from build123d import *

# Parameters (mm, degrees)
BOSS_EXTRUDE1_DEPTH = 280
SKETCH5_W           = 95
SKETCH5_H           = 160
SKETCH5_W_2         = 95.780958046
CUT_EXTRUDE9_DEPTH  = 280
FILLET1_RADIUS      = 30
FILLET1_LENGTH      = 15
FILLET2_RADIUS      = 30
FILLET2_LENGTH      = 15
FILLET3_RADIUS      = 30
FILLET3_LENGTH      = 15
FILLET4_RADIUS      = 30
FILLET4_LENGTH      = 15
SKETCH7_R           = 15
CUT_EXTRUDE10_DEPTH = 280
SKETCH8_W           = 140
SKETCH8_H           = 61.010205144
CUT_EXTRUDE11_DEPTH = 280
FILLET5_RADIUS      = 35
FILLET5_LENGTH      = 15
FILLET6_RADIUS      = 35
FILLET6_LENGTH      = 15
FILLET7_RADIUS      = 35
FILLET7_LENGTH      = 15
FILLET8_RADIUS      = 35
FILLET8_LENGTH      = 15
SKETCH9_R           = 15
CUT_EXTRUDE12_DEPTH = 280


with BuildPart() as part:
    # Sketch1 → Boss-Extrude1 (new body)
    with BuildSketch(Plane.XY):
        with BuildLine():
            Line((-120, -40), (-37.749172176, -40))
            ThreePointArc((-37.749172176, -40), (-54.444104817, 7.799964787), (-25, 48.989794856))
            Line((-25, 48.989794856), (-25, 110))
            Line((-25, 110), (-10, 110))
            Line((-10, 110), (-10, 38.729833462))
            ThreePointArc((-10, 38.729833462), (0, -40), (10, 38.729833462))
            Line((10, 38.729833462), (10, 110))
            Line((10, 110), (25, 110))
            Line((25, 110), (25, 48.989794856))
            ThreePointArc((25, 48.989794856), (54.444104817, 7.799964787), (37.749172176, -40))
            Line((37.749172176, -40), (120, -40))
            Line((120, -40), (120, -55))
            Line((120, -55), (-120, -55))
            Line((-120, -55), (-120, -40))
        make_face()
    extrude(amount=-BOSS_EXTRUDE1_DEPTH)

    # Sketch5 → Cut-Extrude9 (cut)
    with BuildSketch(Plane(origin=(0, -40, 0), x_dir=(1, 0, 0), z_dir=(0, 1, 0))):
        with Locations((72.5, 140)):
            Rectangle(SKETCH5_W, SKETCH5_H)
        with Locations((-72.109520977, 140)):
            Rectangle(SKETCH5_W_2, SKETCH5_H)
    extrude(amount=-CUT_EXTRUDE9_DEPTH, mode=Mode.SUBTRACT)

    # Fillet1: full round fillet: the end face becomes a half cylinder, R = half its width
    fillet1_face = Plane((-120, -47.5, -250), x_dir=(0, -1, 0), z_dir=(-1, 0, 0))  # on the end face: x along it, z out of the body
    fillet1_slab = fillet1_face.offset(-FILLET1_RADIUS / 2) * Box(FILLET1_LENGTH, 2 * FILLET1_RADIUS, FILLET1_RADIUS, mode=Mode.PRIVATE)  # the body's end, R deep
    fillet1_round = Plane((-90, -47.5, -250), x_dir=(-1, 0, 0), z_dir=(0, -1, 0)) * Cylinder(FILLET1_RADIUS, FILLET1_LENGTH, mode=Mode.PRIVATE)  # its axis R under the face
    add(fillet1_slab - fillet1_round, mode=Mode.SUBTRACT)

    # Fillet2: full round fillet: the end face becomes a half cylinder, R = half its width
    fillet2_face = Plane((-120, -47.5, -30), x_dir=(0, 1, 0), z_dir=(-1, 0, 0))  # on the end face: x along it, z out of the body
    fillet2_slab = fillet2_face.offset(-FILLET2_RADIUS / 2) * Box(FILLET2_LENGTH, 2 * FILLET2_RADIUS, FILLET2_RADIUS, mode=Mode.PRIVATE)  # the body's end, R deep
    fillet2_round = Plane((-90, -47.5, -30), x_dir=(-1, 0, 0), z_dir=(0, 1, 0)) * Cylinder(FILLET2_RADIUS, FILLET2_LENGTH, mode=Mode.PRIVATE)  # its axis R under the face
    add(fillet2_slab - fillet2_round, mode=Mode.SUBTRACT)

    # Fillet3: full round fillet: the end face becomes a half cylinder, R = half its width
    fillet3_face = Plane((120, -47.5, -250), x_dir=(0, 1, 0), z_dir=(1, 0, 0))  # on the end face: x along it, z out of the body
    fillet3_slab = fillet3_face.offset(-FILLET3_RADIUS / 2) * Box(FILLET3_LENGTH, 2 * FILLET3_RADIUS, FILLET3_RADIUS, mode=Mode.PRIVATE)  # the body's end, R deep
    fillet3_round = Plane((90, -47.5, -250), x_dir=(1, 0, 0), z_dir=(0, 1, 0)) * Cylinder(FILLET3_RADIUS, FILLET3_LENGTH, mode=Mode.PRIVATE)  # its axis R under the face
    add(fillet3_slab - fillet3_round, mode=Mode.SUBTRACT)

    # Fillet4: full round fillet: the end face becomes a half cylinder, R = half its width
    fillet4_face = Plane((120, -47.5, -30), x_dir=(0, -1, 0), z_dir=(1, 0, 0))  # on the end face: x along it, z out of the body
    fillet4_slab = fillet4_face.offset(-FILLET4_RADIUS / 2) * Box(FILLET4_LENGTH, 2 * FILLET4_RADIUS, FILLET4_RADIUS, mode=Mode.PRIVATE)  # the body's end, R deep
    fillet4_round = Plane((90, -47.5, -30), x_dir=(1, 0, 0), z_dir=(0, -1, 0)) * Cylinder(FILLET4_RADIUS, FILLET4_LENGTH, mode=Mode.PRIVATE)  # its axis R under the face
    add(fillet4_slab - fillet4_round, mode=Mode.SUBTRACT)

    # Sketch7 → Cut-Extrude10 (cut)
    with BuildSketch(Plane(origin=(0, -40, 0), x_dir=(1, 0, 0), z_dir=(0, 1, 0))):
        with Locations(Location((-90, 250, 0), (0, 0, 180))):
            Circle(SKETCH7_R)
        with Locations(Location((90, 250, 0), (0, 0, 180))):
            Circle(SKETCH7_R)
        with Locations(Location((90, 30, 0), (0, 0, 180))):
            Circle(SKETCH7_R)
        with Locations(Location((-90, 30, 0), (0, 0, 180))):
            Circle(SKETCH7_R)
    extrude(amount=-CUT_EXTRUDE10_DEPTH, mode=Mode.SUBTRACT)

    # Sketch8 → Cut-Extrude11 (cut)
    with BuildSketch(Plane(origin=(25, 0, 0), x_dir=(0, 0, -1), z_dir=(1, 0, 0))):
        with Locations((140, 79.494897428)):
            Rectangle(SKETCH8_W, SKETCH8_H)
    extrude(amount=-CUT_EXTRUDE11_DEPTH, mode=Mode.SUBTRACT)

    # Fillet5: full round fillet: the end face becomes a half cylinder, R = half its width
    fillet5_face = Plane((17.5, 110, -35), x_dir=(1, 0, 0), z_dir=(0, 1, 0))  # on the end face: x along it, z out of the body
    fillet5_slab = fillet5_face.offset(-FILLET5_RADIUS / 2) * Box(FILLET5_LENGTH, 2 * FILLET5_RADIUS, FILLET5_RADIUS, mode=Mode.PRIVATE)  # the body's end, R deep
    fillet5_round = Plane((17.5, 75, -35), x_dir=(0, 1, 0), z_dir=(1, 0, 0)) * Cylinder(FILLET5_RADIUS, FILLET5_LENGTH, mode=Mode.PRIVATE)  # its axis R under the face
    add(fillet5_slab - fillet5_round, mode=Mode.SUBTRACT)

    # Fillet6: full round fillet: the end face becomes a half cylinder, R = half its width
    fillet6_face = Plane((-17.5, 110, -35), x_dir=(1, 0, 0), z_dir=(0, 1, 0))  # on the end face: x along it, z out of the body
    fillet6_slab = fillet6_face.offset(-FILLET6_RADIUS / 2) * Box(FILLET6_LENGTH, 2 * FILLET6_RADIUS, FILLET6_RADIUS, mode=Mode.PRIVATE)  # the body's end, R deep
    fillet6_round = Plane((-17.5, 75, -35), x_dir=(0, 1, 0), z_dir=(1, 0, 0)) * Cylinder(FILLET6_RADIUS, FILLET6_LENGTH, mode=Mode.PRIVATE)  # its axis R under the face
    add(fillet6_slab - fillet6_round, mode=Mode.SUBTRACT)

    # Fillet7: full round fillet: the end face becomes a half cylinder, R = half its width
    fillet7_face = Plane((-17.5, 110, -245), x_dir=(1, 0, 0), z_dir=(0, 1, 0))  # on the end face: x along it, z out of the body
    fillet7_slab = fillet7_face.offset(-FILLET7_RADIUS / 2) * Box(FILLET7_LENGTH, 2 * FILLET7_RADIUS, FILLET7_RADIUS, mode=Mode.PRIVATE)  # the body's end, R deep
    fillet7_round = Plane((-17.5, 75, -245), x_dir=(0, 1, 0), z_dir=(1, 0, 0)) * Cylinder(FILLET7_RADIUS, FILLET7_LENGTH, mode=Mode.PRIVATE)  # its axis R under the face
    add(fillet7_slab - fillet7_round, mode=Mode.SUBTRACT)

    # Fillet8: full round fillet: the end face becomes a half cylinder, R = half its width
    fillet8_face = Plane((17.5, 110, -245), x_dir=(1, 0, 0), z_dir=(0, 1, 0))  # on the end face: x along it, z out of the body
    fillet8_slab = fillet8_face.offset(-FILLET8_RADIUS / 2) * Box(FILLET8_LENGTH, 2 * FILLET8_RADIUS, FILLET8_RADIUS, mode=Mode.PRIVATE)  # the body's end, R deep
    fillet8_round = Plane((17.5, 75, -245), x_dir=(0, 1, 0), z_dir=(1, 0, 0)) * Cylinder(FILLET8_RADIUS, FILLET8_LENGTH, mode=Mode.PRIVATE)  # its axis R under the face
    add(fillet8_slab - fillet8_round, mode=Mode.SUBTRACT)

    # Sketch9 → Cut-Extrude12 (cut)
    with BuildSketch(Plane(origin=(25, 0, 0), x_dir=(0, 0, -1), z_dir=(1, 0, 0))):
        with Locations((35, 75)):
            Circle(SKETCH9_R)
        with Locations((245, 75)):
            Circle(SKETCH9_R)
    extrude(amount=-CUT_EXTRUDE12_DEPTH, mode=Mode.SUBTRACT)


solid = part.part
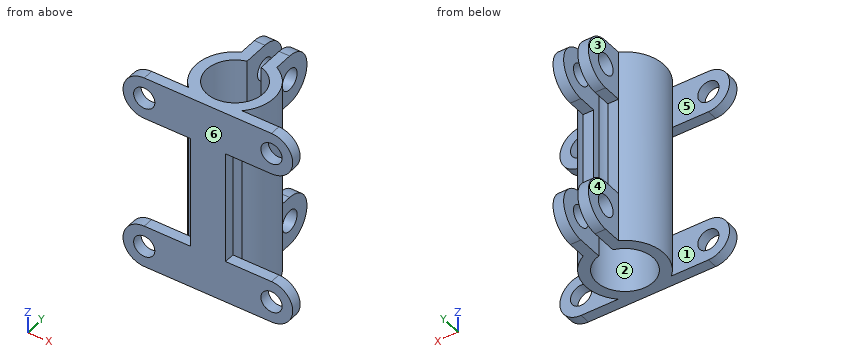
Source: CAD feature listing. Evaluate the final solid. Frame: model axes, mm. Face numbers are marked on the shaded views. A direction names the side the tool comes from. Give positions to 0.01 mm unless a question says otherwise; leave off trailing zeros. Order: outer loops, then holes, each group sorted by start corner. A loop starts at its lowest first (then second) coordinate and runs counter-clockwise, first axis right, second up. Notation, with made-up numbers: (16.25, -7) -> (49.25, -7) arc R14 ccw to (49.25, 3) -> close; hole circle Ø4 at (-22.75, 59.25). An arc over 180 degrees is marked (long way). Write item = value, one per line.
Item 1: Ray query, probe 1 along X at (y, z) = (-47, -248.5); probe 2 along Z at (x, y) = (-90, -47.5); probe 3 along X at (y, z) = (62.5, -265.5). Return the intervals inside material, ascending.
Check result:
probe_1 = -119.96 to -104.92, -75.08 to 75.08, 104.92 to 119.96
probe_2 = -280 to -265, -235 to -220, -60 to -45, -15 to 0
probe_3 = -25 to -10, 10 to 25
Item 2: Section query A-A (y = 0). Output: boundary loops of the cut face in (x, z), then the cut area to 3 significant figures.
Check result:
outline = (-55, -280) -> (-40, -280) -> (-40, 0) -> (-55, 0) -> close; (40, -280) -> (55, -280) -> (55, 0) -> (40, 0) -> close
area = 8,400 mm²
Item 3: Section query B-B (x = -14). Output: boundary loops of the cut face in (y, z), then the cut area to 3 significant figures.
Check result:
outline = (-55, -280) -> (-37.47, -280) -> (-37.47, 0) -> (-55, 0) -> close; (37.47, -280) -> (75, -280) arc R35 ccw to (75, -210) -> (48.99, -210) -> (48.99, -70) -> (75, -70) arc R35 ccw to (75, 0) -> (37.47, 0) -> close; hole circle Ø30 at (75, -245); hole circle Ø30 at (75, -35)
area = 14,200 mm²
Item 4: Contact query for flat-ended pins moving along their axis: pin 1 (24 mm diameter, centred on x = 90, z = -30, fed in from +Y); pin 2 (5 mm diameter, centred on x = 19, y = 90.5, fed in from +Z); pin 3 (18.5 mm diameter, centred on y = 86, z = -254.5, fed in from -X); pin 4 (7 mm diameter, centred on x = -33.5, z = -131, fed in from -Y). Output: stop coordinate, or through.
Check result:
pin_1 = through
pin_2 = -2.5
pin_3 = -25
pin_4 = -40
Item 5: Set-up query: the marked faces 1, 2 and 3. Return all of +Z, -Z, +X, -X, +Y, -Y with unobstructed straight access to the full face (end or side cutting, diameter ignored); none if empty.
Check result:
face_1 = +Z, -Z, -X
face_2 = +Z, -Z
face_3 = +Z, -Z, -X, +Y
Item 6: Section query C-C (z = -250). State how many separate pieces and enclosed holes the cut face has, then the cut area to 3 significant figures.
Check result:
separate_pieces = 5
enclosed_holes = 0
area = 6,980 mm²
Item 7: Mould query, pull axis Y, two halves, no side actions, for the marked faces 4, 5 and 6. Classes: +Y half, -Y half, draft (parallel to the pull), parting line (faces both ways), or undercut.
Check result:
face_4 = draft
face_5 = undercut
face_6 = -Y half
